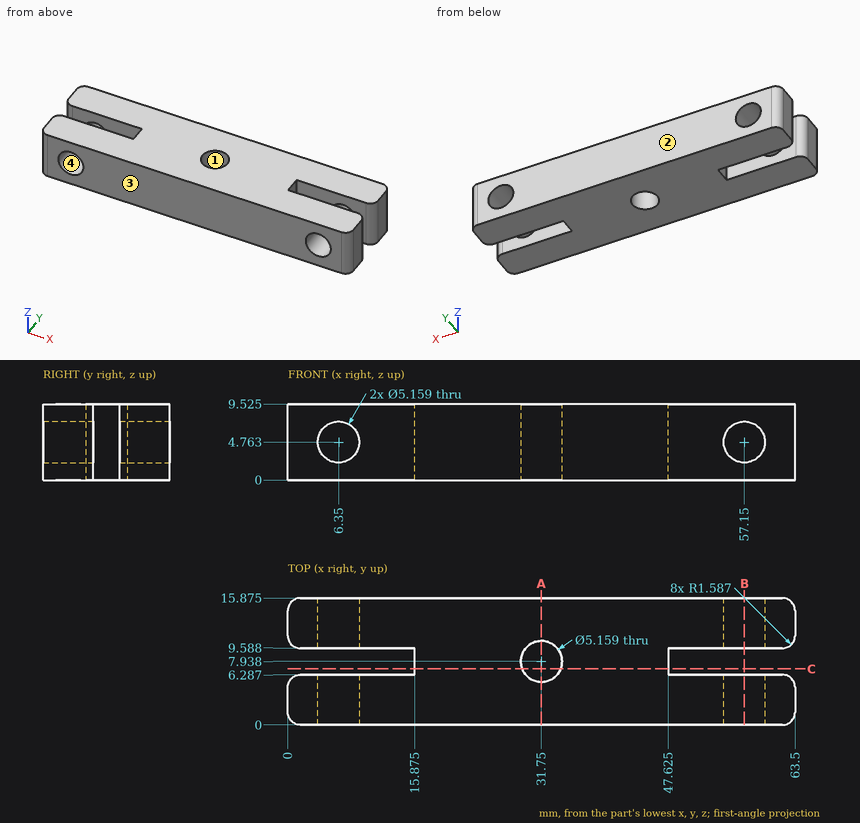
Answer from the drawing. Dimensions are ordinates in mm from the lowest x, y and z of the part. Round coordinates to 2 decimals unless told otherwise and drop trailing zeros. Loops run counter-clockwise (first coordinate to the right, second up) from the corner with the lowest first, then second, coordinate; pieces in that order, holes last.
1) A cutting plane is placed at C-C on y = 7. Determine the outline of the cut face in (x, z) (1 decimal), plus the area to 3 significant figures.
Outcome:
outline: (15.9, 0) - (29.3, 0) - (29.3, 9.5) - (15.9, 9.5) - close; (34.2, 0) - (47.6, 0) - (47.6, 9.5) - (34.2, 9.5) - close
area: 257 mm2
2) A cutting plane is placed at A-A on x = 31.75. Determine the outline of the cut face in (y, z) (1 decimal).
Outcome:
outline: (0, 0) - (5.4, 0) - (5.4, 9.5) - (0, 9.5) - close; (10.5, 0) - (15.9, 0) - (15.9, 9.5) - (10.5, 9.5) - close
3) Given P1, Ø2.5, axis at y = 7, z = 6.5, coming from the -X side; P2, Ø5, axis at y = 8.5, z = 5, coming from the -X side, each flat-ended and moving along its own axis, determine where each tip first touches the part or whether it passes through.
Outcome:
P1: stops at x = 0.4
P2: stops at x = 0.01
4) A cutting plane is placed at B-B on x = 57.15. Determine the outline of the cut face in (y, z) (1 decimal).
Outcome:
outline: (0, 0) - (6.3, 0) - (6.3, 2.2) - (0, 2.2) - close; (0, 7.3) - (6.3, 7.3) - (6.3, 9.5) - (0, 9.5) - close; (9.6, 0) - (15.9, 0) - (15.9, 2.2) - (9.6, 2.2) - close; (9.6, 7.3) - (15.9, 7.3) - (15.9, 9.5) - (9.6, 9.5) - close
5) For a pull along Y with two mould halves and no side action, classify the marked faces 1, 2, 3 and 4 as released by +Y, released by -Y, zero draft, split by the parting line, or undercut.
Outcome:
face 1: undercut
face 2: released by +Y
face 3: released by -Y
face 4: zero draft
6) Consider line 1 (Z direction, x = 57.15, y = 2.75) (1 decimal); line 2 (Y direction, x = 8, z = 8) (1 decimal); line 3 (X direction, y = 10.25, z = 5.5) (1 decimal). Determine where each line is inside the solid, lowest interval first.
Outcome:
line 1: z = 0 to 2.2, 7.3 to 9.5
line 2: y = 0 to 6.3, 9.6 to 15.9
line 3: x = 0.3 to 3.9, 8.8 to 30.6, 32.9 to 54.7, 59.6 to 63.2
